Model file for the job. Use its own axes, mm. Round coordinates to 2 decimals unless told otherwise and drop trailing zeros. Write each loop counter-clockwise with the first axis right and the second up, starting at its lowest first coordinate (ties: lowest second). Pieces come first, ordered by that corner, then holes. Notation, with made-up numbers: (33.5, 40) - (82.5, 40) arc R18 cw to (82.5, 57) - close; hole circle Ø7 at (7.5, 60). An arc over 180 degrees is marked (long way). One line per item, written item: value.
from build123d import *

# Parameters (mm, degrees)
SKETCH_1_R          = 6
SKETCH_1_R_2        = 5
EXTRUDE_1_DEPTH     = 1
CUT_EXTRUDE_1_DEPTH = 1
EXTRUDE_2_DEPTH     = 1


with BuildPart() as part:
    # 草图1 → 凸台-拉伸1 (new body)
    with BuildSketch(Plane.XY):
        Circle(SKETCH_1_R)
        Circle(SKETCH_1_R_2, mode=Mode.SUBTRACT)
    extrude(amount=EXTRUDE_1_DEPTH)

    # 草图2 → 切除-拉伸1 (cut)
    with BuildSketch(Plane.XY.offset(1)):
        Polygon((0, 0), (0, 9.552056019), (-2.79719818, 8.880094398), align=None)
    extrude(amount=-CUT_EXTRUDE_1_DEPTH, mode=Mode.SUBTRACT)

    # 草图3 → 凸台-拉伸2 (add)
    with BuildSketch(Plane.XY.offset(1)):
        Polygon((0, 6), (0, 6.882885988), (0.831959966, 7.145879705), (0.94595308, 6.785271442), (0.314049211, 6.585518144), (0.314049211, 5.991775454), align=None)
        Polygon((-2.099729946, 5.620599092), (-1.80266094, 5.722797702), (-2.067918288, 6.564894019), (-2.940456135, 6.56578037), (-2.940840318, 6.187583858), (-2.278116072, 6.186910643), align=None)
    extrude(amount=-EXTRUDE_2_DEPTH)


solid = part.part
1. Band-saw the part on C-C on z = 0.35. Write the cut outline in (x, y).
Report:
outline: (-2.94, 6.19) - (-2.28, 6.19) - (-2.1, 5.62) arc R6 ccw (long way) to (0.31, 5.99) - (0.31, 6.59) - (0.95, 6.79) - (0.83, 7.15) - (0, 6.88) - (0, 5) arc R5 cw (long way) to (-1.5, 4.77) - (-2.07, 6.56) - (-2.94, 6.57) - close
2. Band-saw the part on B-B on x = -3.75. Write the cut outline in (y, z), plus the area to 3 significant figures.
Report:
outline: (-4.68, 0) - (-3.31, 0) - (-3.31, 1) - (-4.68, 1) - close; (3.31, 0) - (4.68, 0) - (4.68, 1) - (3.31, 1) - close
area: 2.75 mm²
3. Band-saw the part on A-A on y = 0. Write the cut outline in (x, z).
Report:
outline: (-6, 0) - (-5, 0) - (-5, 1) - (-6, 1) - close; (5, 0) - (6, 0) - (6, 1) - (5, 1) - close
4. Wall check: probe 1 along X at (y, z) = (0, 0.45); probe 2 along Y at (x, z) = (-2.75, 0.1); probe 3 along Y at (x, z) = (-2.5, 0.4). Give the ranges that are in metal, low to high. Write a range as [from, to].
Report:
probe 1: [-6, -5], [5, 6]
probe 2: [-5.33, -4.18], [4.18, 5.33], [6.19, 6.57]
probe 3: [-5.45, -4.33], [4.33, 5.45], [6.19, 6.57]
5. Drop a flat-ended pin along its axis: pin 1 (6 mm diameter, centred on x = 3, y = 1, fed in from +Z). Give the stop position or say it passes through.
Report:
pin 1: z = 1
6. Band-saw the part on D-D on x = -1.25. Write the cut outline in (y, z), plus the area to 3 significant figures.
Report:
outline: (-5.87, 0) - (-4.84, 0) - (-4.84, 1) - (-5.87, 1) - close
area: 1.03 mm²
7. Mould opens along Y. For faces 1 (the face through (0, 5.9, 0.5)), 2 (the face through (0.41, 7.013, 0.507)), 3 (the face through (0.55, -4.97, 0.49)) say: released by +Y, released by -Y, zero draft, split by the parting line, or undercut.
Report:
face 1: zero draft
face 2: released by +Y
face 3: undercut
